from build123d import *

# Parameters (mm, degrees)
SKETCH1_W           = 58.7375
SKETCH1_H           = 104.775
SKETCH1_W_2         = 52.3875
SKETCH1_H_2         = 98.425
EXTRUDE_THIN1_DEPTH = 38.1
FILLET1_R           = 3.175
BOSS_EXTRUDE1_DEPTH = 3.175
FILLET2_R           = 3.175
SKETCH3_R           = 2.06375
CUT_EXTRUDE1_DEPTH  = 3.175
CIRPATTERN1_COUNT   = 2
FILLET3_R           = 1.5875


with BuildPart() as part:
    # Sketch1 → Extrude-Thin1 (new body)
    with BuildSketch(Plane(origin=(0, 0, 0), x_dir=(1, 0, 0), z_dir=(0, 1, 0))):
        Rectangle(SKETCH1_W, SKETCH1_H)
        Rectangle(SKETCH1_W_2, SKETCH1_H_2, mode=Mode.SUBTRACT)
    extrude(amount=EXTRUDE_THIN1_DEPTH)

    # Fillet1
    fillet1_edges = [part.edges().sort_by_distance(p)[0] for p in [
        (26.19375, 19.05, 49.2125),
        (26.19375, 19.05, -49.2125),
        (-26.19375, 19.05, -49.2125),
        (-26.19375, 19.05, 49.2125),
        (29.36875, 19.05, 52.3875),
        (-29.36875, 19.05, 52.3875),
        (-29.36875, 19.05, -52.3875),
        (29.36875, 19.05, -52.3875),
    ]]
    fillet(fillet1_edges, radius=FILLET1_R)

    # Sketch2 → Boss-Extrude1 (add)
    with BuildSketch(Plane.XZ):
        with BuildLine():
            Line((29.36875, -49.2125), (29.36875, 49.2125))
            ThreePointArc((29.36875, 49.2125), (28.43881403, 51.45756403), (26.19375, 52.3875))
            Line((26.19375, 52.3875), (-26.19375, 52.3875))
            ThreePointArc((-26.19375, 52.3875), (-28.43881403, 51.45756403), (-29.36875, 49.2125))
            Line((-29.36875, 49.2125), (-29.36875, -49.2125))
            ThreePointArc((-29.36875, -49.2125), (-28.43881403, -51.45756403), (-26.19375, -52.3875))
            Line((-26.19375, -52.3875), (26.19375, -52.3875))
            ThreePointArc((26.19375, -52.3875), (28.43881403, -51.45756403), (29.36875, -49.2125))
        make_face()
    extrude(amount=BOSS_EXTRUDE1_DEPTH)

    # Fillet2
    fillet2_edges = [part.edges().sort_by_distance(p)[0] for p in [
        (26.19375, 0, 0),
        (0, 0, -49.2125),
        (-26.19375, 0, 0),
        (0, 0, 49.2125),
        (-25.26381403, 0, 48.28256403),
        (25.26381403, 0, 48.28256403),
        (25.26381403, 0, -48.28256403),
        (-25.26381403, 0, -48.28256403),
    ]]
    fillet(fillet2_edges, radius=FILLET2_R)

    # Sketch3 → Cut-Extrude1 (cut)
    with BuildSketch(Plane(origin=(0, 0, 0), x_dir=(1, 0, 0), z_dir=(0, 1, 0))):
        with Locations(Location((-16.66875, 39.6875, 0), (0, 0, 270))):
            Circle(SKETCH3_R)
    cut_extrude1 = extrude(amount=-CUT_EXTRUDE1_DEPTH, mode=Mode.SUBTRACT)

    # Sketch4 → Cut-Revolve1 (revolve, cut)
    with BuildSketch(Plane.YX.offset(39.6875), mode=Mode.PRIVATE) as cut_revolve1_sk:
        Polygon((-2.480052205, -16.66875), (0, -12.54125), (0, -16.66875), align=None)
    cut_revolve1 = revolve(cut_revolve1_sk.sketch.rotate(Axis((-16.66875, 0, -39.6875), (0, -1, 0)), 90), axis=Axis((-16.66875, 0, -39.6875), (0, -1, 0)), mode=Mode.SUBTRACT)

    # CirPattern1: Cut-Extrude1, Cut-Revolve1 ×2 about axis
    cirpattern1_axis = Axis((0, 0, 0), (0, 1, 0))
    add([cut_extrude1.rotate(cirpattern1_axis, i * 360 / CIRPATTERN1_COUNT) for i in range(1, CIRPATTERN1_COUNT)], mode=Mode.SUBTRACT)
    add([cut_revolve1.rotate(cirpattern1_axis, i * 360 / CIRPATTERN1_COUNT) for i in range(1, CIRPATTERN1_COUNT)], mode=Mode.SUBTRACT)

    # Fillet3
    fillet3_edges = [part.edges().sort_by_distance(p)[0] for p in [
        (29.36875, 38.1, 0),
        (0, 38.1, 52.3875),
        (0, 38.1, -52.3875),
        (-29.36875, 38.1, 0),
        (0, 38.1, -49.2125),
        (26.19375, 38.1, 0),
        (0, 38.1, 49.2125),
        (-26.19375, 38.1, 0),
        (-28.43881403, 38.1, 51.45756403),
        (28.43881403, 38.1, -51.45756403),
        (-28.43881403, 38.1, -51.45756403),
        (28.43881403, 38.1, 51.45756403),
        (-25.26381403, 38.1, 48.28256403),
        (25.26381403, 38.1, 48.28256403),
        (25.26381403, 38.1, -48.28256403),
        (-25.26381403, 38.1, -48.28256403),
    ]]
    fillet(fillet3_edges, radius=FILLET3_R - 0.0001)  # a hair under: the kernel refuses the full size


solid = part.part
Here's how the part is built. I have some questions about the finished solid (model axes, mm). A direction names the side the tool comes from. Give positions to 0.01 mm unless a question says otherwise; leave off trailing zeros. Answer as a JSON object with one key per item and string values. Group by question number.
Item 1: Will these pins go through, and if not, where does the flat tip stop? pin 1 (2 mm diameter, centred on x = 4, z = 41, fed in from +Y); pin 2 (3.5 mm diameter, centred on x = 16.67, z = 39.69, fed in from -Y).
Item 2: Thinking about a two-plate mould opening in X: for faces 3 (the flat face through (29.369, 17, -1)), 4 (the cylindrical face through (-25.239, 20.077, -48.307)), 5 (the flat face through (0, 17, 52.388)), which applies, pulls with the +X half, pulls with the -X half, needs draft (parallel to the pull), parting line crosses it, or undercut?
Item 3: On a 3-axis mill with a long thin cutter (end or side, diameter ignored), from which of +Z, -Z, +X, -X, +Y, -Y can I reach the whole of each face in a straight line? I mean faces 1 (the flat face through (-26.194, 20, 1)), 2 (the flat face through (-29.369, 17, 1)). Say none if no direction works.
Item 4: I need wall thicknesses on L1, parallel to Z at x = 8.5, y = 26; L2, parallel to X at y = 26, z = 20; L3, parallel to Y at x = -3.5, z = -38.5 (3 decimals). Which ranges of each line are inside material? Lowest first, please.
Answer list:
{
 "1": {"pin 1": "stops at y = 0", "pin 2": "passes through"},
 "2": {"face 3": "pulls with the +X half", "face 4": "undercut", "face 5": "needs draft"},
 "3": {"face 1": "+Y", "face 2": "+Z, -Z, -X, +Y, -Y"},
 "4": {"L1": "z = -52.39 to -49.21, 49.21 to 52.39", "L2": "x = -29.37 to -26.19, 26.19 to 29.37", "L3": "y = -3.175 to 0"}
}
